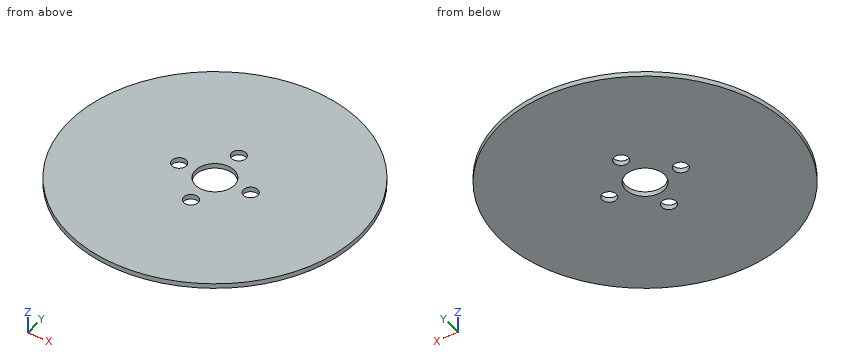
Autodesk Inventor part; units mm, degrees
ref_plane "YZ Plane" through (0, 0, 0) normal (1, 0, 0) x (0, 1, 0)
ref_plane "XZ Plane" through (0, 0, 0) normal (0, 1, 0) x (-1, 0, 0)
ref_plane "XY Plane" through (0, 0, 0) normal (0, 0, 1) x (1, 0, 0)
sketch "Sketch1" plane through (0, 0, 0) normal (0, 0, 1) x (1, 0, 0)
  circle A0 centre (0, 0) radius 30
  dimension "d0" = 60
extrude "Extrusion1" add sketch "Sketch1" along normal mid plane 1
sketch "Sketch2" plane through (0, 0, 0.5) normal (0, 0, 1) x (1, 0, 0)
  point P0 (0, 0)
  point P1 (0, 0)
hole "Hole1" at (0, 0, 0.5) direction (0, 0, -1) diameter 8 end through all
sketch "Sketch3" plane through (0, 0, 0.5) normal (0, 0, 1) x (1, 0, 0)
  circle A0 centre (0, 0) radius 4
  circle A1 centre (0, 0) radius 7.5 construction
  point P0 (-7.5, 0)
  point P1 (0, 7.5)
  point P2 (7.5, 0)
  point P3 (0, -7.5)
  dimension "d10" = 15
hole "Hole2" at (-7.5, 0, 0.5) at (0, 7.5, 0.5) at (7.5, 0, 0.5) at (0, -7.5, 0.5) direction (0, 0, -1) diameter 3 end through all
properties part number "plate" material "Steel"
Check sheet for the modelled part. Datum: model origin and axes. Units: mm. Give positions to 0.01 mm unless a question says otherwise; leave off trailing zeros. Loops run counter-clockwise (first coordinate to the right, second up) from the corner with the lowest first, then second, coordinate; pieces in that order, holes last. Notation, with made-up numbers: M 71.25,-4.75 L 103.25,-4.75 A21 cw 103.25,9.25 Z; hole C -5,-19 d10. An arc over 180 degrees is marked long. Use a Markdown table: item, result. Add a question column.
Q1. Sectioned sample at C-C, the plane y = 7.5. Record the cut outline in (x, z), then the cut area to 3 significant figures.
Q2. Sectioned sample at B-B, the plane z = -0.1. Record the cut outline in (x, y), then the cut area to 3 significant figures.
Q3. Sectioned sample at A-A, the plane x = 0. Record the cut outline in (y, z), then the cut area to 3 significant figures.
Q4. Scan lines: line 1 along Y through (x, z) = (0, -0.05); line 2 along Y through (x, z) = (7, 0.25); line 3 along Y through (x, z) = (-7.5, -0.15). Record each from-to range of solid material in increasing order. Write a range as [from, to].
Verdict:
| question | item | result |
|---|---|---|
| 1 | outline | M -29.05,-0.5 L -1.5,-0.5 L -1.5,0.5 L -29.05,0.5 Z; M 1.5,-0.5 L 29.05,-0.5 L 29.05,0.5 L 1.5,0.5 Z |
| 1 | area | 55.1 mm^2 |
| 2 | outline | C 0,0 d60; hole C -7.5,0 d3; hole C 0,0 d8; hole C 0,-7.5 d3; hole C 0,7.5 d3; hole C 7.5,0 d3 |
| 2 | area | 2,750 mm^2 |
| 3 | outline | M -30,-0.5 L -9,-0.5 L -9,0.5 L -30,0.5 Z; M -6,-0.5 L -4,-0.5 L -4,0.5 L -6,0.5 Z; M 4,-0.5 L 6,-0.5 L 6,0.5 L 4,0.5 Z; M 9,-0.5 L 30,-0.5 L 30,0.5 L 9,0.5 Z |
| 3 | area | 46.0 mm^2 |
| 4 | line 1 | [-30, -9], [-6, -4], [4, 6], [9, 30] |
| 4 | line 2 | [-29.17, -1.41], [1.41, 29.17] |
| 4 | line 3 | [-29.05, -1.5], [1.5, 29.05] |
